from build123d import *

# Parameters (mm, degrees)
BOSS_EXTRUDE1_DEPTH             = 2.6
SKETCH5_W                       = 11.826356456
SKETCH5_H                       = 5.621169426
CUT_EXTRUDE2_DEPTH              = 7.632050589
SKETCH6_W                       = 11.690711404
SKETCH6_H                       = 7.254613366
CUT_EXTRUDE3_DEPTH              = 5.2
SKETCH7_W                       = 0.5
SKETCH7_H                       = 0.5
BOSS_EXTRUDE2_DEPTH             = 12.7
BOSS_EXTRUDE2_DIRECTION_2_REACH = 8.542
SKETCH8_R                       = 0.8
CUT_EXTRUDE4_DEPTH              = 0.2
SKETCH10_W                      = 6.769382977
SKETCH10_H                      = 8.778669798
CUT_EXTRUDE5_DEPTH              = 17.078911904


with BuildPart() as part:
    # Sketch2 → Boss-Extrude1 (new, symmetric)
    with BuildSketch(Plane(origin=(0, 0, 0), x_dir=(1, 0, 0), z_dir=(0, 1, 0))):
        with BuildLine():
            Line((-2.105447518, 1.212026432), (2.105447518, 1.212026432))
            ThreePointArc((2.105447518, 1.212026432), (0, -2.977973568), (-2.105447518, 1.212026432))
        make_face()
    extrude(amount=BOSS_EXTRUDE1_DEPTH, both=True)

    # Sketch5 → Cut-Extrude2 (cut, through all)
    with BuildSketch(Plane(origin=(0, 2.580250079, -0.225742631), x_dir=(1, 0, 0), z_dir=(0, 0.9961946980917455, -0.08715574274765836))):
        with Locations((0.924694538, -0.744658901)):
            Rectangle(SKETCH5_W, SKETCH5_H)
    cut_extrude2 = extrude(amount=CUT_EXTRUDE2_DEPTH, mode=Mode.SUBTRACT)

    # Sketch6 → Cut-Extrude3 (cut)
    with BuildSketch(Plane(origin=(0, 2.580250079, 0.225742631), x_dir=(1, 0, 0), z_dir=(0, 0.9961946980917467, 0.08715574274764504))):
        with Locations((0.257342704, -2.465539164)):
            Rectangle(SKETCH6_W, SKETCH6_H)
    cut_extrude3 = extrude(amount=CUT_EXTRUDE3_DEPTH, mode=Mode.SUBTRACT)

    # Mirror1: Cut-Extrude2, Cut-Extrude3 across plane
    add(cut_extrude2.mirror(Plane.ZX), mode=Mode.SUBTRACT)
    add(cut_extrude3.mirror(Plane.ZX), mode=Mode.SUBTRACT)

    # Sketch7 → Boss-Extrude2 (add)
    with BuildSketch(Plane(origin=(0, -2.6, 0), x_dir=(-1, 0, 0), z_dir=(0, -1, 0))):
        with Locations((-1.27, 0.25)):
            Rectangle(SKETCH7_W, SKETCH7_H)
        with Locations((0, 0.25)):
            Rectangle(SKETCH7_W, SKETCH7_H)
        with Locations((1.27, 0.25)):
            Rectangle(SKETCH7_W, SKETCH7_H)
    extrude(amount=BOSS_EXTRUDE2_DEPTH)

    # Sketch7 → Boss-Extrude2 direction 2 (add, up to next)
    with BuildSketch(Plane(origin=(0, -2.6, 0), x_dir=(-1, 0, 0), z_dir=(0, -1, 0)), mode=Mode.PRIVATE) as boss_extrude2_direction_2_sk1:
        with Locations((-1.27, 0.25)):
            Rectangle(SKETCH7_W, SKETCH7_H)
    boss_extrude2_direction_2_tool1 = extrude(boss_extrude2_direction_2_sk1.sketch, amount=-BOSS_EXTRUDE2_DIRECTION_2_REACH, mode=Mode.PRIVATE) - part.part
    # Sketch7 → Boss-Extrude2 direction 2 (add, up to next)
    with BuildSketch(Plane(origin=(0, -2.6, 0), x_dir=(-1, 0, 0), z_dir=(0, -1, 0)), mode=Mode.PRIVATE) as boss_extrude2_direction_2_sk2:
        with Locations((0, 0.25)):
            Rectangle(SKETCH7_W, SKETCH7_H)
    boss_extrude2_direction_2_tool2 = extrude(boss_extrude2_direction_2_sk2.sketch, amount=-BOSS_EXTRUDE2_DIRECTION_2_REACH, mode=Mode.PRIVATE) - part.part
    # Sketch7 → Boss-Extrude2 direction 2 (add, up to next)
    with BuildSketch(Plane(origin=(0, -2.6, 0), x_dir=(-1, 0, 0), z_dir=(0, -1, 0)), mode=Mode.PRIVATE) as boss_extrude2_direction_2_sk3:
        with Locations((1.27, 0.25)):
            Rectangle(SKETCH7_W, SKETCH7_H)
    boss_extrude2_direction_2_tool3 = extrude(boss_extrude2_direction_2_sk3.sketch, amount=-BOSS_EXTRUDE2_DIRECTION_2_REACH, mode=Mode.PRIVATE) - part.part
    add(boss_extrude2_direction_2_tool1.solids().sort_by_distance((1.27, -2.6, -0.25))[0])
    add(boss_extrude2_direction_2_tool2.solids().sort_by_distance((0, -2.6, -0.25))[0])
    add(boss_extrude2_direction_2_tool3.solids().sort_by_distance((-1.27, -2.6, -0.25))[0])

    # Sketch8 → Cut-Extrude4 (cut)
    with BuildSketch(Plane.XY.offset(2.977973568)):
        Circle(SKETCH8_R)
    extrude(amount=-CUT_EXTRUDE4_DEPTH, mode=Mode.SUBTRACT)

    # Sketch10 → Cut-Extrude5 (cut, through all)
    with BuildSketch(Plane(origin=(0, 0, -1.212026432), x_dir=(-1, 0, 0), z_dir=(0, 0, -1))):
        with Locations((0.550161867, -12.189334899)):
            Rectangle(SKETCH10_W, SKETCH10_H)
    extrude(amount=-CUT_EXTRUDE5_DEPTH, mode=Mode.SUBTRACT)


solid = part.part
Input: part model. Units: mm. Frame: model coordinates. Round coordinates to 2 decimals unless told otherwise and drop trailing zeros. Loops run counter-clockwise (first coordinate to the right, second up) from the corner with the lowest first, then second, coordinate; pieces in that order, holes last. Notation, with made-up numbers: (13.5, 1) -> (56.5, 1) arc R20 ccw to (56.5, 28) -> close; hole circle Ø8 at (82, -25.75). An arc over 180 degrees is marked (long way). Answer as a JSON object with one key per item and string values. Group by question number.
1) Draft query along Y for faces 1 (the flat face through (0, 0, -1.212)), 2 (the flat face through (0, 0, 2.778)), 3 (the flat face through (-0.04, -2.5, 1.14)), 4 (the flat face through (-0.04, 2.5, 1.14)). Return one class per face: +Y half, -Y half, draft (parallel to the pull), parting line (faces both ways), or undercut.
2) Section query C-C on z = -0.15. Output: boundary loops of the cut face in (x, y), plus the area to 3 significant figures.
3) Section query A-A on y = -6.5. Output: boundary loops of the cut face in (x, z).
4) Pin query (flat end, axial travel): pin 1 (1.3 mm diameter, centred on x = 0, y = 0, fed in from +Z); pin 2 (0.6 mm diameter, centred on y = -6, z = -0.5, fed in from +X); pin 3 (0.6 mm diameter, centred on x = -1, y = -5.5, fed in from -Z). Return the tip coordinate at first contact, or that it passes through.
5) Section query B-B on x = 0. Output: boundary loops of the cut face in (y, z), plus the area to 3 significant figures.
6) Ray query, L1, parallel to X at y = -6.25, z = -0.4; L2, parallel to Y at x = -0.9, z = 1.2; L3, parallel to Y at x = 0, z = 2.9. Return the intervals inside material, ascending.
7) Section query D-D on y = 0. Output: boundary loops of the cut face in (x, z).
Reply:
{
 "1": {"face 1": "draft", "face 2": "undercut", "face 3": "-Y half", "face 4": "+Y half"},
 "2": {"outline": "(-2.58, -2.59) -> (-1.52, -2.59) -> (-1.52, -7.8) -> (-1.02, -7.8) -> (-1.02, -2.59) -> (-0.25, -2.59) -> (-0.25, -7.8) -> (0.25, -7.8) -> (0.25, -2.59) -> (1.02, -2.59) -> (1.02, -7.8) -> (1.52, -7.8) -> (1.52, -2.59) -> (2.58, -2.59) -> (2.58, 2.59) -> (-2.58, 2.59) -> close", "area": "34.5 mm2"},
 "3": {"outline": "(-1.52, -0.5) -> (-1.02, -0.5) -> (-1.02, 0) -> (-1.52, 0) -> close; (-0.25, -0.5) -> (0.25, -0.5) -> (0.25, 0) -> (-0.25, 0) -> close; (1.02, -0.5) -> (1.52, -0.5) -> (1.52, 0) -> (1.02, 0) -> close"},
 "4": {"pin 1": "stops at z = 2.78", "pin 2": "stops at x = 1.52", "pin 3": "stops at z = -0.5"},
 "5": {"outline": "(-7.8, -0.5) -> (-2.56, -0.5) -> (-2.49, -1.21) -> (2.49, -1.21) -> (2.6, 0) -> (2.34, 2.98) -> (0.8, 2.98) -> (0.8, 2.78) -> (-0.8, 2.78) -> (-0.8, 2.98) -> (-2.34, 2.98) -> (-2.6, 0) -> (-7.8, 0) -> close", "area": "23.2 mm2"},
 "6": {"L1": "x = -1.52 to -1.02, -0.25 to 0.25, 1.02 to 1.52", "L2": "y = -2.5 to 2.5", "L3": "y = -2.35 to -0.8, 0.8 to 2.35"},
 "7": {"outline": "(-2.11, -1.21) -> (2.11, -1.21) arc R2.62 ccw to (0.8, 2.85) -> (0.8, 2.78) -> (-0.8, 2.78) -> (-0.8, 2.85) arc R2.62 ccw to start"}
}
